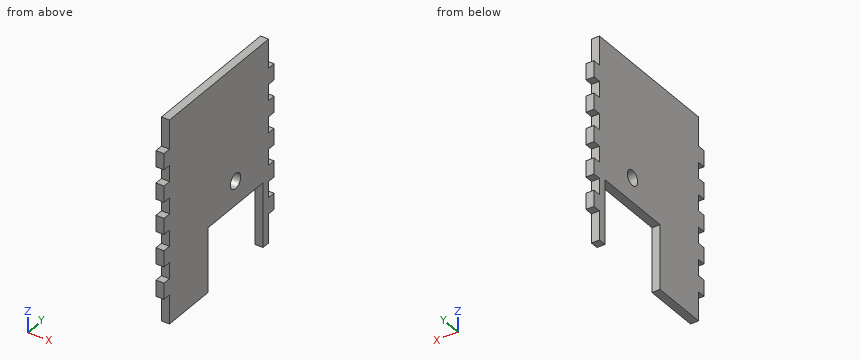
```python
from build123d import *

# Parameters (mm, degrees)
SKETCH2_W           = 80.01
SKETCH2_H           = 63.5
BOSS_EXTRUDE1_DEPTH = 3.175
SKETCH3_W           = 11.43
SKETCH3_H           = 3.175
SKETCH3_W_2         = 6.35
CUT_EXTRUDE1_DEPTH  = 4.175
SKETCH4_R           = 2.9845
SKETCH4_W           = 25.4
SKETCH4_H           = 31.75
CUT_EXTRUDE2_DEPTH  = 4.175


with BuildPart() as part:
    # Sketch2 → Boss-Extrude1 (new body)
    with BuildSketch(Plane(origin=(0, 0, 0), x_dir=(0, 0, -1), z_dir=(1, 0, 0))):
        Rectangle(SKETCH2_W, SKETCH2_H)
    extrude(amount=BOSS_EXTRUDE1_DEPTH)

    # Sketch3 → Cut-Extrude1 (cut, through all)
    with BuildSketch(Plane.ZY):
        with Locations((-34.29, -30.1625)):
            Rectangle(SKETCH3_W, SKETCH3_H)
        with Locations((-19.05, -30.1625)):
            Rectangle(SKETCH3_W_2, SKETCH3_H)
        with Locations((-6.35, -30.1625)):
            Rectangle(SKETCH3_W_2, SKETCH3_H)
        with Locations((6.35, -30.1625)):
            Rectangle(SKETCH3_W_2, SKETCH3_H)
        with Locations((19.05, -30.1625)):
            Rectangle(SKETCH3_W_2, SKETCH3_H)
        with Locations((34.29, -30.1625)):
            Rectangle(SKETCH3_W, SKETCH3_H)
        with Locations((34.29, 30.1625)):
            Rectangle(SKETCH3_W, SKETCH3_H)
        with Locations((19.05, 30.1625)):
            Rectangle(SKETCH3_W_2, SKETCH3_H)
        with Locations((6.35, 30.1625)):
            Rectangle(SKETCH3_W_2, SKETCH3_H)
        with Locations((-6.35, 30.1625)):
            Rectangle(SKETCH3_W_2, SKETCH3_H)
        with Locations((-19.05, 30.1625)):
            Rectangle(SKETCH3_W_2, SKETCH3_H)
        with Locations((-34.29, 30.1625)):
            Rectangle(SKETCH3_W, SKETCH3_H)
    extrude(amount=-CUT_EXTRUDE1_DEPTH, mode=Mode.SUBTRACT)

    # Sketch4 → Cut-Extrude2 (cut, through all)
    with BuildSketch(Plane(origin=(3.175, 0, 0), x_dir=(0, 0, -1), z_dir=(1, 0, 0))):
        with Locations((5.08, 9.525)):
            Circle(SKETCH4_R)
        with Locations((27.305, 9.525)):
            Rectangle(SKETCH4_W, SKETCH4_H)
    extrude(amount=-CUT_EXTRUDE2_DEPTH, mode=Mode.SUBTRACT)


solid = part.part
```
The model under review builds one solid part; all positions refer to its coordinate system, in mm. Give positions to 0.01 mm unless a question says otherwise; leave off trailing zeros. Write each loop counter-clockwise with the first axis right and the second up, starting at its lowest first coordinate (ties: lowest second). Pieces come first, ordered by that corner, then holes. Notation, with made-up numbers: (3.25, -40) -> (26.25, -40) arc R14 ccw to (26.25, -33) -> close; hole circle Ø1 at (-28, 34). An arc over 180 degrees is marked (long way). Put each result on its own line as item: value.
(1) We need section D-D, the plane z = 29.5. Give the boundary of the cut face in (x, y) (3 decimals).
Results are:
outline: (0, -28.575) -> (3.175, -28.575) -> (3.175, 28.575) -> (0, 28.575) -> close
(2) We need section C-C, the plane y = 17. Give the boundary of the cut face in (x, z) (3 decimals), and give its area (3 significant figures).
Results are:
outline: (0, -14.605) -> (3.175, -14.605) -> (3.175, 40.005) -> (0, 40.005) -> close
area: 173 mm²
(3) For pin 1 Ø1 at (x, y) = (2.5, 29.5) entering from +Z (3 decimals); pin 2 Ø1 at (x, y) = (2.5, -30) entering from -Z (3 decimals); pin 3 Ø1 at (x, z) = (2, 34) entering from +Y (3 decimals), all flat-tipped, find the tip position at first contact; note any pin that passes through.
Results are:
pin 1: z = 28.575
pin 2: z = -28.575
pin 3: y = 28.575
(4) We need section A-A, the plane z = -27.5. Give the boundary of the cut face in (x, y) (3 decimals).
Results are:
outline: (0, -31.75) -> (3.175, -31.75) -> (3.175, -6.35) -> (0, -6.35) -> close; (0, 25.4) -> (3.175, 25.4) -> (3.175, 31.75) -> (0, 31.75) -> close
(5) We need section B-B, the plane z = -17.5. Give the boundary of the cut face in (x, y) (3 decimals).
Results are:
outline: (0, -28.575) -> (3.175, -28.575) -> (3.175, -6.35) -> (0, -6.35) -> close; (0, 25.4) -> (3.175, 25.4) -> (3.175, 28.575) -> (0, 28.575) -> close
(6) To check wall thickness, follow probe 1 along Y at (x, z) = (2, -5.08) (1 decimal); probe 2 along Y at (x, z) = (2.9, -28.5); probe 3 along Y at (x, z) = (1.6, 33) (3 decimals). State the ranges of each line that lie inside material, in increasing order. Write a range as from..to.
Results are:
probe 1: -28.6..6.5, 12.5..28.6
probe 2: -31.75..-6.35, 25.4..31.75
probe 3: -28.575..28.575
